Geometry check sheet. Reference: the model listing, model coordinates, mm. A direction names the side the tool comes from. Round coordinates to 2 decimals unless told otherwise and drop trailing zeros. Order: outer loops, then holes, each group sorted by start corner. A loop starts at its lowest first (then second) coordinate and runs counter-clockwise, first axis right, second up. Notation, with made-up numbers: (48, 9) -> (107, 9) arc R22 cw to (107, 25) -> close; hole circle Ø1 at (87.5, 68). An arc over 180 degrees is marked (long way). Use a Markdown table: item, result. Add a question column.
Item 1: Sectioned sample at C-C, the plane z = 25. State how many separate pieces and enclosed holes the cut face has, and give its area (3 significant figures).
Item 2: Material ranges on probe 1 along Z at (x, y) = (4, -54); probe 2 along X at (y, z) = (-44.5, 15); probe 3 along Y at (x, z) = (6, 28.5), recorded low to high. Write a range as [from, to].
Item 3: Sectioned sample at D-D, the plane z = 21.5. Record the cut outline in (x, y).
Item 4: Sectioned sample at B-B, the plane x = 52. Record the cut outline in (y, z).
Item 5: Sectioned sample at A-A, the plane y = -47. Record the cut outline in (x, z).
Item 6: Gauge pin test, flat end, axial feed: pin 1 Ø3 at (x, y) = (15.5, -41.5) entering from +Z. Record the tip position at first contact, or that the pin passes through.
Item 7: Mould release check, pull along Z, two halves, no side actions. Record for faces 4 (the flat face through (8, -49, 20)), 5 (the cylindrical face through (50.8, -48.8, 14.1)), 6 (the flat face through (28, -30, 10)), 7 (the cylindrical face through (5.386, -48.846, 14.425)): pulls with the +Z half, pulls with the -Z half, needs draft (parallel to the pull), parting line crosses it, or undercut.
Item 8: Set-up check for faces 1 (the flat face through (8, -11, 20)), 2 (the flat face through (28, -60, 8)), 3 (the flat face through (52, -38, 20)): record each of +Z, -Z, +X, -X, +Y, -Y from which the full face is reachable in a straight line by a thin tool's end or side.
from build123d import *

# Parameters (mm, degrees)
CYLINDER003_R     = 1.5
CYLINDER003_DEPTH = 60
CYLINDER002_R     = 1.5
CYLINDER002_DEPTH = 60
CYLINDER001_R     = 1.5
CYLINDER001_DEPTH = 60
CYLINDER_R        = 1.5
CYLINDER_DEPTH    = 60
SKETCH_W          = 56.05
SKETCH_H          = 60
PAD_DEPTH         = 10
SKETCH003_W       = 8
SKETCH003_H       = 22
PAD002_DEPTH      = 30
SKETCH004_W       = 8
SKETCH004_H       = 22
PAD003_DEPTH      = 30
SKETCH005_W       = 8
SKETCH005_H       = 22
PAD004_DEPTH      = 30
SKETCH006_W       = 8
SKETCH006_H       = 22
PAD005_DEPTH      = 30


with BuildPart() as cylinder003:
    # Cylinder003 → Cylinder003 (new body)
    with BuildSketch(Plane(origin=(52, 0, 15), x_dir=(1, 0, 0), z_dir=(0, -1, 0))):
        Circle(CYLINDER003_R)
    extrude(amount=CYLINDER003_DEPTH)


with BuildPart() as cylinder002:
    # Cylinder002 → Cylinder002 (new body)
    with BuildSketch(Plane(origin=(52, 0, 25), x_dir=(1, 0, 0), z_dir=(0, -1, 0))):
        Circle(CYLINDER002_R)
    extrude(amount=CYLINDER002_DEPTH)


with BuildPart() as cylinder001:
    # Cylinder001 → Cylinder001 (new body)
    with BuildSketch(Plane(origin=(4, 0, 15), x_dir=(1, 0, 0), z_dir=(0, -1, 0))):
        Circle(CYLINDER001_R)
    extrude(amount=CYLINDER001_DEPTH)


with BuildPart() as cylinder:
    # Cylinder → Cylinder (new body)
    with BuildSketch(Plane(origin=(4, 0, 25), x_dir=(1, 0, 0), z_dir=(0, -1, 0))):
        Circle(CYLINDER_R)
    extrude(amount=CYLINDER_DEPTH)


with BuildPart() as cut003:
    # Sketch → Pad (new body)
    with BuildSketch(Plane.XY):
        with Locations((28.025, -30)):
            Rectangle(SKETCH_W, SKETCH_H)
    extrude(amount=PAD_DEPTH)

    # Sketch003 → Pad002 (join)
    with BuildSketch(Plane.XY):
        with Locations((4, -11)):
            Rectangle(SKETCH003_W, SKETCH003_H)
    extrude(amount=PAD002_DEPTH)

    # Sketch004 → Pad003 (join)
    with BuildSketch(Plane.XY):
        with Locations((52.05, -11)):
            Rectangle(SKETCH004_W, SKETCH004_H)
    extrude(amount=PAD003_DEPTH)

    # Sketch005 → Pad004 (join)
    with BuildSketch(Plane.XY):
        with Locations((4, -49)):
            Rectangle(SKETCH005_W, SKETCH005_H)
    extrude(amount=PAD004_DEPTH)

    # Sketch006 → Pad005 (join)
    with BuildSketch(Plane.XY):
        with Locations((52.05, -49)):
            Rectangle(SKETCH006_W, SKETCH006_H)
    extrude(amount=PAD005_DEPTH)

    # Cut: cut Cylinder
    add(cylinder.part, mode=Mode.SUBTRACT)

    # Cut001: cut Cylinder001
    add(cylinder001.part, mode=Mode.SUBTRACT)

    # Cut002: cut Cylinder002
    add(cylinder002.part, mode=Mode.SUBTRACT)

    # Cut003: cut Cylinder003
    add(cylinder003.part, mode=Mode.SUBTRACT)


solid = cut003.part
Found:
| question | item | result |
|---|---|---|
| 1 | separate pieces | 8 |
| 1 | enclosed holes | 0 |
| 1 | area | 440 mm2 |
| 2 | probe 1 | z = [0, 13.5], [16.5, 23.5], [26.5, 30] |
| 2 | probe 2 | x = [0, 2.5], [5.5, 8], [48.05, 50.5], [53.5, 56.05] |
| 2 | probe 3 | y = [-60, -38], [-22, 0] |
| 3 | outline | (0, -60) -> (8, -60) -> (8, -38) -> (0, -38) -> close; (0, -22) -> (8, -22) -> (8, 0) -> (0, 0) -> close; (48.05, -60) -> (56.05, -60) -> (56.05, -38) -> (48.05, -38) -> close; (48.05, -22) -> (56.05, -22) -> (56.05, 0) -> (48.05, 0) -> close |
| 4 | outline | (-60, 0) -> (0, 0) -> (0, 13.5) -> (-22, 13.5) -> (-22, 10) -> (-38, 10) -> (-38, 13.5) -> (-60, 13.5) -> close; (-60, 16.5) -> (-38, 16.5) -> (-38, 23.5) -> (-60, 23.5) -> close; (-60, 26.5) -> (-38, 26.5) -> (-38, 30) -> (-60, 30) -> close; (-22, 16.5) -> (0, 16.5) -> (0, 23.5) -> (-22, 23.5) -> close; (-22, 26.5) -> (0, 26.5) -> (0, 30) -> (-22, 30) -> close |
| 5 | outline | (0, 0) -> (56.05, 0) -> (56.05, 30) -> (48.05, 30) -> (48.05, 10) -> (8, 10) -> (8, 30) -> (0, 30) -> close; hole circle Ø3 at (4, 15); hole circle Ø3 at (4, 25); hole circle Ø3 at (52, 15); hole circle Ø3 at (52, 25) |
| 6 | pin 1 | stops at z = 10 |
| 7 | face 4 | needs draft |
| 7 | face 5 | undercut |
| 7 | face 6 | pulls with the +Z half |
| 7 | face 7 | undercut |
| 8 | face 1 | +Z, +Y, -Y |
| 8 | face 2 | +Z, -Z, +X, -X, -Y |
| 8 | face 3 | +Z, +X, -X |
